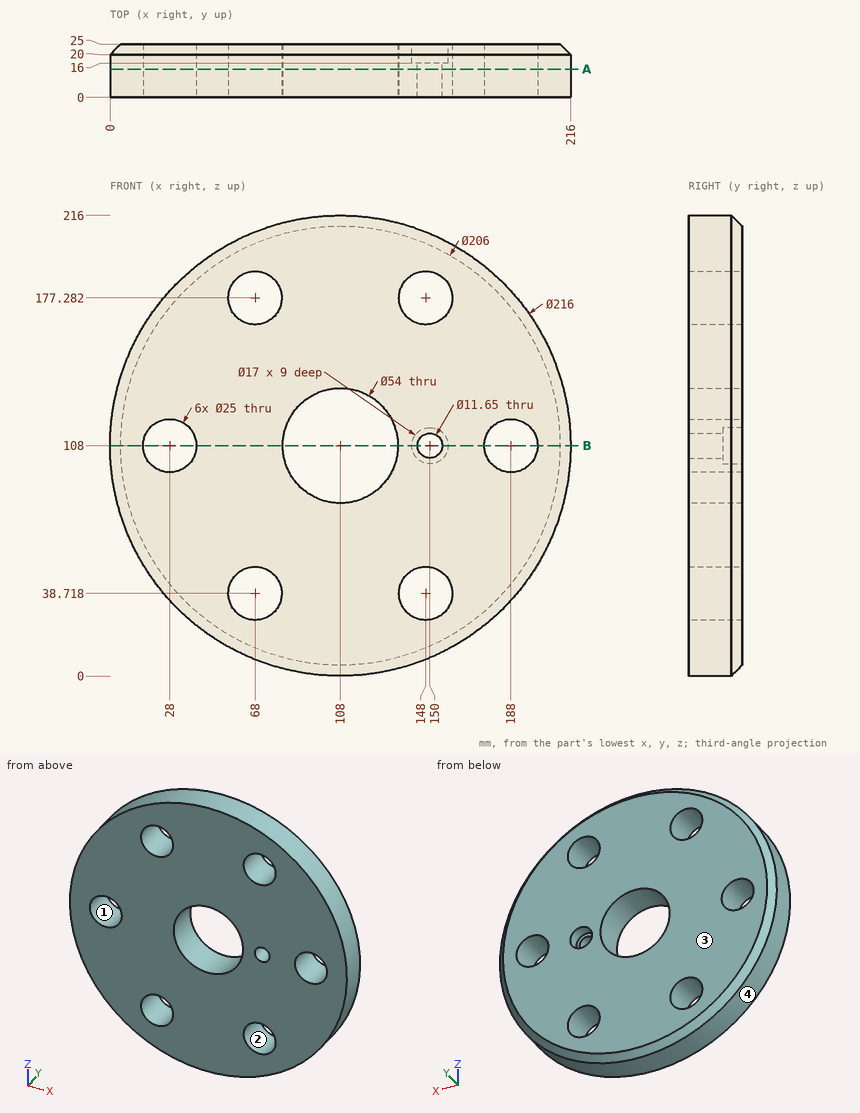
Could you check a few things on this drawing? It's one solid part, dimensions in mm from its lowest x, y, z. Round coordinates to 2 decimals unless told otherwise and drop trailing zeros. Loops run counter-clockwise (first coordinate to the right, second up) from the corner with the lowest first, then second, coordinate; pieces in that order, holes last. Notation, with made-up numbers: M -22,37 L -4,37 A13 ccw -4,50 Z; hole C 50,63.5 d8. An arc over 180 degrees is marked long. Write item = value, one per line. Start each with the question number.
(1) Suppose I cut it at B-B on z = 108. Write out the boundary of the cut face in (x, y) (3 decimals), plus the area to 3 significant figures.
(2) I need wall thicknesses on line 1 along X through (y, z) = (16, 44.5); line 2 along X through (y, z) = (6.75, 172.5); line 3 along X through (y, z) = (8, 107). Which ranges of each line are inside material? Lowest first, please.
(3) I'm going to push flat-ended pins straight in: P1, Ø3, axis at y = 3.5, z = 84.5, coming from the +X side; P2, Ø22.5, axis at x = 188, z = 108, coming from the -Y side; P3, Ø10, axis at x = 156, y = 11, coming from the -Z side; P4, Ø15.5, axis at x = 150, z = 108, coming from the +Y side. Where does each tip first touch, or does it pass through?
(4) Suppose I cut it at A-A on y = 13.25. Give the number of separate pieces and of enclosed holes in the cut face, plus the area to 3 significant figures.
(5) If we mould it in two halves opening along X, with no side actions, what happens to the marked faces 1, 2, 3 and 4? For each: released by +X, released by -X, zero draft, split by the parting line, or undercut.
Answer block:
q1.outline = M 0,0 L 15.5,0 L 15.5,25 L 5,25 L 0,20 Z; M 40.5,0 L 81,0 L 81,25 L 40.5,25 Z; M 135,0 L 144.175,0 L 144.175,16 L 141.5,16 L 141.5,25 L 135,25 Z; M 155.825,0 L 175.5,0 L 175.5,25 L 158.5,25 L 158.5,16 L 155.825,16 Z; M 200.5,0 L 216,0 L 216,20 L 211,25 L 200.5,25 Z
q1.area = 2,440 mm²
q2.line_1 = 20.64 to 56.92, 79.08 to 136.92, 159.08 to 195.36
q2.line_2 = 21.38 to 56.45, 79.55 to 136.45, 159.55 to 194.62
q2.line_3 = 0 to 15.54, 40.46 to 81.02, 134.98 to 144.26, 155.74 to 175.54, 200.46 to 216
q3.P1 = 213.74
q3.P2 = through
q3.P3 = 8.93
q3.P4 = 16
q4.separate_pieces = 1
q4.enclosed_holes = 8
q4.area = 31,300 mm²
q5.face_1 = undercut
q5.face_2 = undercut
q5.face_3 = zero draft
q5.face_4 = split by the parting line
